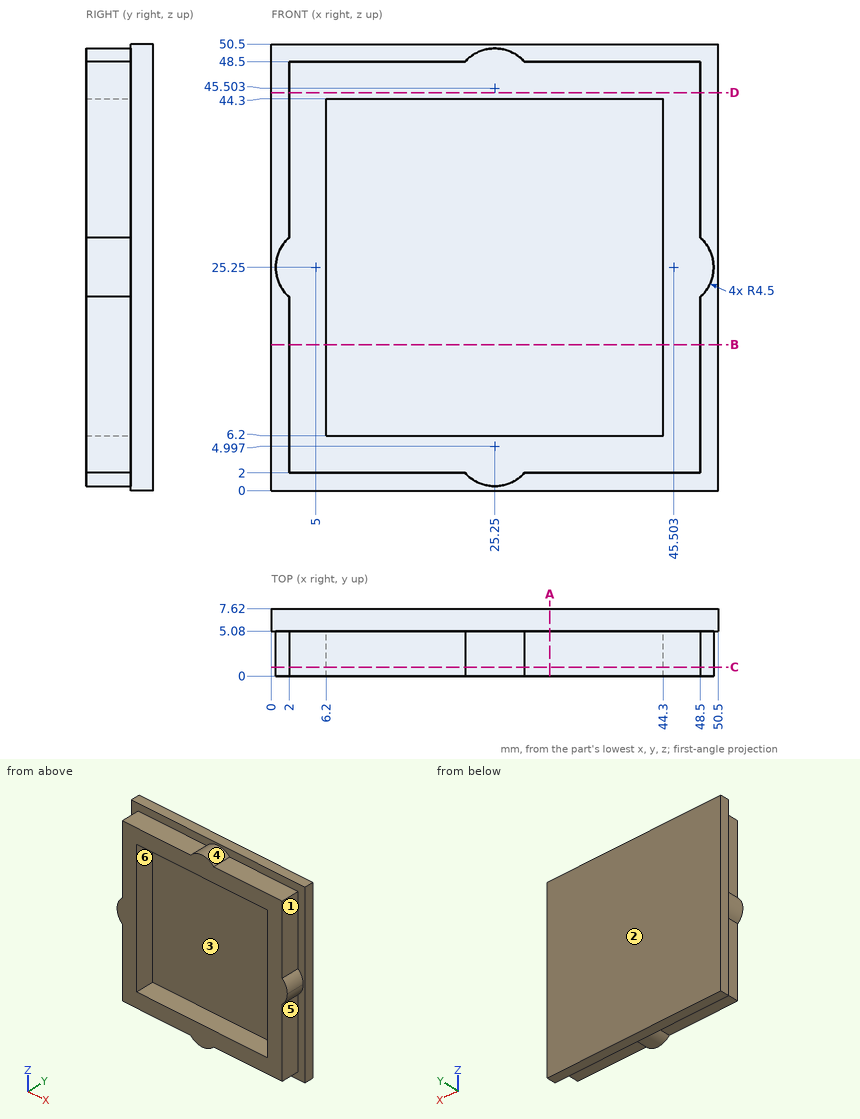
Print and shaded views of the part. All mm, measured from the part's lowest x, y and z. A direction names the side the tool comes from. Coordinates: 2 decimals unless noted, no trailing zeros. Write each loop counter-clockwise with the first axis right and the second up, starting at its lowest first coordinate (ties: lowest second). Pieces come first, ordered by that corner, then holes.
(1) Cut at B-B, the plane z = 16.5. List the corners of the cut face in (x, y), and give its area (3 significant figures).
(2) Two-plate mould, pull along Z, no slides. Class the marked faces 4, 5 and 6: +Z half, -Z half, draft (parallel to the pull), parting line (faces both ways), or undercut.
(3) Drill centre lines: probe 1 along Z at (x, y) = (19, 2.25); probe 2 along X at (y, z) = (4.5, 4). Where is each one in solid material? Low to high.
(4) Cut at C-C, the plane y = 1. List the corners of the cut face in (x, z).
(5) 3-axis set-ups, long thin cutter, end or side, ignore diameter. For the marked faces 1, 2 and 3: which of +Z, -Z, +X, -X, +Y, -Y reach the whole face in a straight line?
(6) Flat gauge pins, fed straight in: pin 1 (4 mm diameter, centred on x = 38.5, y = 2, fed in from +Z); pin 2 (2.5 mm diameter, centred on y = 1.5, z = 43, fed in from -X); pin 3 (2 mm diameter, centred on x = 39, z = 32.5, fed in from -Y). Where does each tip first touch, or does it go through?
(7) Cut at A-A, the plane x = 31.5. List the corners of the cut face in (y, z), and give its area (3 significant figures).
(8) Cut at D-D, the plane z = 45. List the corners of the cut face in (x, y).
Geometry says:
1. outline: (0, 5.08) - (2, 5.08) - (2, 0) - (6.2, 0) - (6.2, 5.08) - (44.3, 5.08) - (44.3, 0) - (48.5, 0) - (48.5, 5.08) - (50.5, 5.08) - (50.5, 7.62) - (0, 7.62) - close
1. area: 171 mm2
2. face 4: +Z half
2. face 5: draft
2. face 6: undercut
3. probe 1: z = 2 to 6.2, 44.3 to 48.5
3. probe 2: x = 2 to 48.5
4. outline: (2, 2) - (21.89, 2) arc R4.5 ccw to (28.61, 2) - (48.5, 2) - (48.5, 21.89) arc R4.5 ccw to (48.5, 28.61) - (48.5, 48.5) - (28.61, 48.5) arc R4.5 ccw to (21.89, 48.5) - (2, 48.5) - (2, 28.6) arc R4.5 ccw to (2, 21.9) - close; hole (6.2, 6.2) - (44.3, 6.2) - (44.3, 44.3) - (6.2, 44.3) - close
5. face 1: +Z, +X, -Y
5. face 2: +Z, -Z, +X, -X, +Y
5. face 3: -Y
6. pin 1: stops at z = 48.5
6. pin 2: stops at x = 2
6. pin 3: stops at y = 5.08
7. outline: (0, 2) - (5.08, 2) - (5.08, 0) - (7.62, 0) - (7.62, 50.5) - (5.08, 50.5) - (5.08, 48.5) - (0, 48.5) - (0, 44.3) - (5.08, 44.3) - (5.08, 6.2) - (0, 6.2) - close
7. area: 171 mm2
8. outline: (0, 5.08) - (2, 5.08) - (2, 0) - (48.5, 0) - (48.5, 5.08) - (50.5, 5.08) - (50.5, 7.62) - (0, 7.62) - close
